from build123d import *

# Parameters (mm, degrees)
BOSS_EXTRUDE1_DEPTH      = 250
BOSS_EXTRUDE1_DEPTH_BACK = 250
SKETCH2_R                = 500
SKETCH3_R                = 490
CUT_EXTRUDE4_DEPTH       = 10
SKETCH5_R                = 478
CUT_EXTRUDE5_DEPTH       = 15
SKETCH6_R                = 100
BOSS_EXTRUDE2_DEPTH      = 10
SKETCH7_R                = 85
BOSS_EXTRUDE3_DEPTH      = 20
SKETCH8_R                = 72
CUT_EXTRUDE6_DEPTH       = 20
FILLET2_R                = 10
SKETCH9_W                = 276.167171278
SKETCH9_H                = 73.496102034
BOSS_EXTRUDE4_DEPTH      = 40
FILLET3_R                = 10
FILLET4_R                = 10
FILLET5_R                = 10
BOSS_EXTRUDE5_START      = 10
SKETCH10_R               = 100
BOSS_EXTRUDE5_DEPTH      = 10
SCALE1_SCALE             = 0.7


# Some blends are built 0.0001 mm under size
with BuildPart() as part:
    # Sketch2 → Boss-Extrude1 (new, two sides: drawn at the far end of the back side and taken through both)
    with BuildSketch(Plane.XY.offset(-BOSS_EXTRUDE1_DEPTH_BACK)):
        Circle(SKETCH2_R)
    extrude(amount=BOSS_EXTRUDE1_DEPTH + BOSS_EXTRUDE1_DEPTH_BACK)

    # Sketch3 → Cut-Extrude4 (cut)
    with BuildSketch(Plane.XY.offset(250)):
        Circle(SKETCH3_R)
    extrude(amount=-CUT_EXTRUDE4_DEPTH, mode=Mode.SUBTRACT)

    # Sketch5 → Cut-Extrude5 (cut)
    with BuildSketch(Plane.XY.offset(240)):
        Circle(SKETCH5_R)
    extrude(amount=-CUT_EXTRUDE5_DEPTH, mode=Mode.SUBTRACT)

    # Sketch6 → Boss-Extrude2 (add)
    with BuildSketch(Plane.XY.offset(225)):
        Circle(SKETCH6_R)
    extrude(amount=BOSS_EXTRUDE2_DEPTH)

    # Sketch7 → Boss-Extrude3 (add)
    with BuildSketch(Plane.XY.offset(235)):
        Circle(SKETCH7_R)
    extrude(amount=BOSS_EXTRUDE3_DEPTH)

    # Sketch8 → Cut-Extrude6 (cut)
    with BuildSketch(Plane.XY.offset(255)):
        Circle(SKETCH8_R)
    extrude(amount=-CUT_EXTRUDE6_DEPTH, mode=Mode.SUBTRACT)

    # Fillet2
    fillet2_edges = [part.edges().sort_by_distance(p)[0] for p in [
        (-85, 0, 235),
    ]]
    fillet(fillet2_edges, radius=FILLET2_R)

    # Sketch9 → Boss-Extrude4 (add)
    with BuildSketch(Plane.XY.offset(220)):
        Rectangle(SKETCH9_W, SKETCH9_H)
    extrude(amount=BOSS_EXTRUDE4_DEPTH)

    # Fillet3
    # the kernel refuses this fillet: 10 mm, written as the material it takes off along each edge
    with BuildSketch(Plane(origin=(128.083585639, -26.748051017, 250), x_dir=(0, 0, 1), z_dir=(1, 0, 0))) as fillet3_piece_1_section:
        Polygon((0, 0), (FILLET3_R * 1.02, 0), (FILLET3_R * 1.02, FILLET3_R * 1.02), (0, FILLET3_R * 1.02), align=None)
    fillet3_piece_1 = extrude(amount=FILLET3_R * 1.02, mode=Mode.PRIVATE)
    fillet3_piece_1 = fillet3_piece_1 - Plane(origin=(128.083585639, -26.748051017, 250), x_dir=(0, 0.7071067811865475, -0.7071067811865475), z_dir=(1, 0, 0)) * Sphere(FILLET3_R, mode=Mode.PRIVATE)
    add(fillet3_piece_1, mode=Mode.SUBTRACT)
    with BuildSketch(Plane(origin=(-128.083585639, -26.748051017, 250), x_dir=(-1, 0, 0), z_dir=(0, 0, 1))) as fillet3_piece_2_section:
        Polygon((0, 0), (FILLET3_R * 1.02, 0), (FILLET3_R * 1.02, FILLET3_R * 1.02), (0, FILLET3_R * 1.02), align=None)
    fillet3_piece_2 = extrude(amount=FILLET3_R * 1.02, mode=Mode.PRIVATE)
    fillet3_piece_2 = fillet3_piece_2 - Plane(origin=(-128.083585639, -26.748051017, 250), x_dir=(0.7071067811865475, 0.7071067811865475, 0), z_dir=(0, 0, 1)) * Sphere(FILLET3_R, mode=Mode.PRIVATE)
    add(fillet3_piece_2, mode=Mode.SUBTRACT)
    with BuildSketch(Plane(origin=(-128.083585639, 26.748051017, 250), x_dir=(0, 0, 1), z_dir=(0, 1, 0))) as fillet3_piece_3_section:
        Polygon((0, 0), (FILLET3_R * 1.02, 0), (FILLET3_R * 1.02, -FILLET3_R * 1.02), (0, -FILLET3_R * 1.02), align=None)
    fillet3_piece_3 = extrude(amount=FILLET3_R * 1.02, mode=Mode.PRIVATE)
    fillet3_piece_3 = fillet3_piece_3 - Plane(origin=(-128.083585639, 26.748051017, 250), x_dir=(0.7071067811865475, 0, -0.7071067811865475), z_dir=(0, 1, 0)) * Sphere(FILLET3_R, mode=Mode.PRIVATE)
    add(fillet3_piece_3, mode=Mode.SUBTRACT)
    with BuildSketch(Plane(origin=(128.083585639, 26.748051017, 250), x_dir=(0, 1, 0), z_dir=(1, 0, 0))) as fillet3_piece_4_section:
        Polygon((0, 0), (FILLET3_R * 1.02, 0), (FILLET3_R * 1.02, FILLET3_R * 1.02), (0, FILLET3_R * 1.02), align=None)
    fillet3_piece_4 = extrude(amount=FILLET3_R * 1.02, mode=Mode.PRIVATE)
    fillet3_piece_4 = fillet3_piece_4 - Plane(origin=(128.083585639, 26.748051017, 250), x_dir=(0, -0.7071067811865475, -0.7071067811865475), z_dir=(1, 0, 0)) * Sphere(FILLET3_R, mode=Mode.PRIVATE)
    add(fillet3_piece_4, mode=Mode.SUBTRACT)
    with BuildSketch(Plane(origin=(128.083585639, -36.748051017, 260), x_dir=(0, 1, 0), z_dir=(-1, 0, 0))) as fillet3_piece_5_section:
        with BuildLine():
            CenterArc((FILLET3_R, FILLET3_R), FILLET3_R, 180, 90)
            Line((0, FILLET3_R), (0, 0))
            Line((0, 0), (FILLET3_R, 0))
        make_face()
    fillet3_piece_5 = extrude(amount=256.167171277, mode=Mode.PRIVATE)
    fillet3_piece_5 = split(fillet3_piece_5, bisect_by=Plane(origin=(102.906545957, -34.337396915, 255), z_dir=(0, 0, 1)), keep=Keep.TOP, mode=Mode.PRIVATE)
    add(fillet3_piece_5, mode=Mode.SUBTRACT)
    with BuildSketch(Plane(origin=(128.083585639, -36.748051017, 260), x_dir=(0, 1, 0), z_dir=(-1, 0, 0))) as fillet3_piece_6_section:
        with BuildLine():
            CenterArc((FILLET3_R, FILLET3_R), FILLET3_R, 180, 90)
            Line((0, FILLET3_R), (0, 0))
            Line((0, 0), (FILLET3_R, 0))
        make_face()
    fillet3_piece_6 = extrude(amount=256.167171277, mode=Mode.PRIVATE)
    fillet3_piece_6 = fillet3_piece_6 - Plane(origin=(0, 0, 253.76582848), x_dir=(1, 0, 0), z_dir=(0, 0, -1)) * Cylinder(85, 553, mode=Mode.PRIVATE)
    add(fillet3_piece_6, mode=Mode.SUBTRACT)
    with BuildSketch(Plane(origin=(128.083585639, -36.748051017, 260), x_dir=(0, 1, 0), z_dir=(-1, 0, 0))) as fillet3_piece_7_section:
        with BuildLine():
            CenterArc((FILLET3_R, FILLET3_R), FILLET3_R, 180, 90)
            Line((0, FILLET3_R), (0, 0))
            Line((0, 0), (FILLET3_R, 0))
        make_face()
    fillet3_piece_7 = extrude(amount=256.167171277, mode=Mode.PRIVATE)
    fillet3_piece_7 = fillet3_piece_7 & Plane(origin=(0, 0, 253.76892881), x_dir=(1, 0, 0), z_dir=(0, 0, 1)) * Cylinder(72, 553, mode=Mode.PRIVATE)
    add(fillet3_piece_7, mode=Mode.SUBTRACT)
    with BuildSketch(Plane(origin=(-138.083585639, -26.748051017, 260), x_dir=(1, 0, 0), z_dir=(0, 1, 0))) as fillet3_piece_8:
        with BuildLine():
            CenterArc((FILLET3_R, FILLET3_R), FILLET3_R, 180, 90)
            Line((0, FILLET3_R), (0, 0))
            Line((0, 0), (FILLET3_R, 0))
        make_face()
    extrude(amount=53.496102033, mode=Mode.SUBTRACT)
    with BuildSketch(Plane(origin=(-128.083585639, 36.748051017, 260), x_dir=(0, 0, -1), z_dir=(1, 0, 0))) as fillet3_piece_9_section:
        with BuildLine():
            CenterArc((FILLET3_R, -FILLET3_R), FILLET3_R, 90, 90)
            Line((0, -FILLET3_R), (0, 0))
            Line((0, 0), (FILLET3_R, 0))
        make_face()
    fillet3_piece_9 = extrude(amount=256.167171277, mode=Mode.PRIVATE)
    fillet3_piece_9 = fillet3_piece_9 - Plane(origin=(0, 0, 253.76582848), x_dir=(1, 0, 0), z_dir=(0, 0, -1)) * Cylinder(85, 553, mode=Mode.PRIVATE)
    add(fillet3_piece_9, mode=Mode.SUBTRACT)
    with BuildSketch(Plane(origin=(-128.083585639, 36.748051017, 260), x_dir=(0, 0, -1), z_dir=(1, 0, 0))) as fillet3_piece_10_section:
        with BuildLine():
            CenterArc((FILLET3_R, -FILLET3_R), FILLET3_R, 90, 90)
            Line((0, -FILLET3_R), (0, 0))
            Line((0, 0), (FILLET3_R, 0))
        make_face()
    fillet3_piece_10 = extrude(amount=256.167171277, mode=Mode.PRIVATE)
    fillet3_piece_10 = split(fillet3_piece_10, bisect_by=Plane(origin=(-70.492794496, 34.331084629, 255), z_dir=(0, 0, 1)), keep=Keep.TOP, mode=Mode.PRIVATE)
    add(fillet3_piece_10, mode=Mode.SUBTRACT)
    with BuildSketch(Plane(origin=(-128.083585639, 36.748051017, 260), x_dir=(0, 0, -1), z_dir=(1, 0, 0))) as fillet3_piece_11_section:
        with BuildLine():
            CenterArc((FILLET3_R, -FILLET3_R), FILLET3_R, 90, 90)
            Line((0, -FILLET3_R), (0, 0))
            Line((0, 0), (FILLET3_R, 0))
        make_face()
    fillet3_piece_11 = extrude(amount=256.167171277, mode=Mode.PRIVATE)
    fillet3_piece_11 = fillet3_piece_11 & Plane(origin=(0, 0, 253.768928808), x_dir=(1, 0, 0), z_dir=(0, 0, 1)) * Cylinder(72, 553, mode=Mode.PRIVATE)
    add(fillet3_piece_11, mode=Mode.SUBTRACT)
    with BuildSketch(Plane(origin=(138.083585639, 26.748051017, 260), x_dir=(0, 0, -1), z_dir=(0, -1, 0))) as fillet3_piece_12:
        with BuildLine():
            CenterArc((FILLET3_R, -FILLET3_R), FILLET3_R, 90, 90)
            Line((0, -FILLET3_R), (0, 0))
            Line((0, 0), (FILLET3_R, 0))
        make_face()
    extrude(amount=53.496102033, mode=Mode.SUBTRACT)
    with BuildSketch(Plane(origin=(138.083585639, 36.748051017, 225), x_dir=(-1, 0, 0), z_dir=(0, 0, 1)), Plane(origin=(138.083585639, -36.748051017, 225), x_dir=(0, 1, 0), z_dir=(0, 0, 1))) as fillet3_piece_13:
        with BuildLine():
            CenterArc((FILLET3_R, FILLET3_R), FILLET3_R, 180, 90)
            Line((0, FILLET3_R), (0, 0))
            Line((0, 0), (FILLET3_R, 0))
        make_face()
    extrude(amount=25, mode=Mode.SUBTRACT)
    with BuildSketch(Plane(origin=(-138.083585639, -36.748051017, 225), x_dir=(0, 1, 0), z_dir=(0, 0, 1)), Plane(origin=(-138.083585639, 36.748051017, 225), x_dir=(1, 0, 0), z_dir=(0, 0, 1))) as fillet3_piece_14:
        with BuildLine():
            CenterArc((FILLET3_R, -FILLET3_R), FILLET3_R, 90, 90)
            Line((0, -FILLET3_R), (0, 0))
            Line((0, 0), (FILLET3_R, 0))
        make_face()
    extrude(amount=25, mode=Mode.SUBTRACT)

    # Fillet4
    fillet4_edges = [part.edges().sort_by_distance(p)[0] for p in [
        (0, 100, 225),
    ]]
    fillet(fillet4_edges, radius=FILLET4_R - 0.0001)  # a hair under: the kernel refuses the full size

    # Fillet5
    fillet5_edges = [part.edges().sort_by_distance(p)[0] for p in [
        (-490, 0, 240),
    ]]
    fillet(fillet5_edges, radius=FILLET5_R - 0.0001)  # a hair under: the kernel refuses the full size

    # Sketch10 → Boss-Extrude5 (add)
    with BuildSketch(Plane(origin=(0, 0, -250), x_dir=(-1, 0, 0), z_dir=(0, 0, -1)).offset(BOSS_EXTRUDE5_START)):
        with Locations(Location((0, 0, 0), (0, 0, 180))):
            Circle(SKETCH10_R)
    extrude(amount=-BOSS_EXTRUDE5_DEPTH)


with BuildPart() as part_1:
    # Scale1: scaled about (0, 0.001114487, -11.134314022)
    add(part.part.scale(SCALE1_SCALE).moved(Location((0, 0.000334346, -3.340294207))))


solid = part_1.part
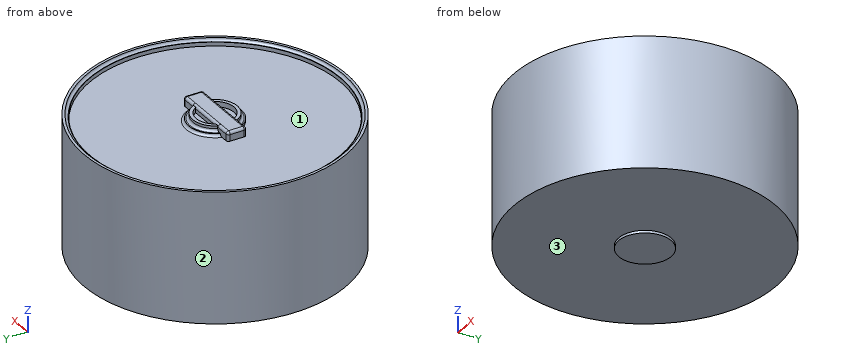
Read the model definition and answer for the solid it produces. Units are mm, in the model's axes. Face numbers are marked on the shaded views. Coordinates: 2 decimals unless noted, no trailing zeros. Loops run counter-clockwise (first coordinate to the right, second up) from the corner with the lowest first, then second, coordinate; pieces in that order, holes last. Notation, with made-up numbers: (13, 62) -> (26, 62) arc R13 ccw to (26, 81) -> close; hole circle Ø11 at (-18.5, 17.5). An arc over 180 degrees is marked (long way). Write item = value, one per line. Start each with the question number.
1) The mould has two halves that part along Y. Classify the marked faces 1, 2 and 3: pulls with the +Y half, pulls with the -Y half, needs draft (parallel to the pull), parting line crosses it, or undercut.
2) The part is cut by section A-A, the plane z = 62. Determine the outline of the cut face in (x, y), plus the area to 3 significant figures.
3) Given P1, Ø22, axis at x = 26.5, y = 54, coming from the +Z side; P2, Ø5.5, axis at x = -73.5, z = 162.5, coming from the -Y side; P3, Ø10, axis at y = 44, z = 21, coming from the -X side, each flat-ended and moving along its own axis, determine where each tip first touches the part or whether it passes through.
4) Find the intervals of material crossed by L1, parallel to Y at x = 0, z = 171.7; L2, parallel to Y at x = 0, z = 162.5; L3, parallel to Z at x = 180, y = -140.5, in increasing order. Write a range as from..to.
Result:
q1.face_1 = undercut
q1.face_2 = parting line crosses it
q1.face_3 = needs draft
q2.outline = circle Ø700 at (0, 0)
q2.area = 385,000 mm²
q3.P1 = 175.16
q3.P2 = -342.77
q3.P3 = -347.82
q4.L1 = -59.5..-50.4, -25.72..25.72, 50.4..59.5
q4.L2 = -350..-334.6, -62.38..-50.4, -25.72..25.72, 50.4..62.38, 334.6..350
q4.L3 = -178.34..154.16
